Check sheet for the drawn part. Datum: minimum x, y, z corner. Units: mm. Give positions to 0.01 mm unless a question says otherwise; leave off trailing zeros. Order: outer loops, then holes, each group sorted by start corner. A loop starts at its lowest first (then second) coordinate and runs counter-clockwise, first axis right, second up.
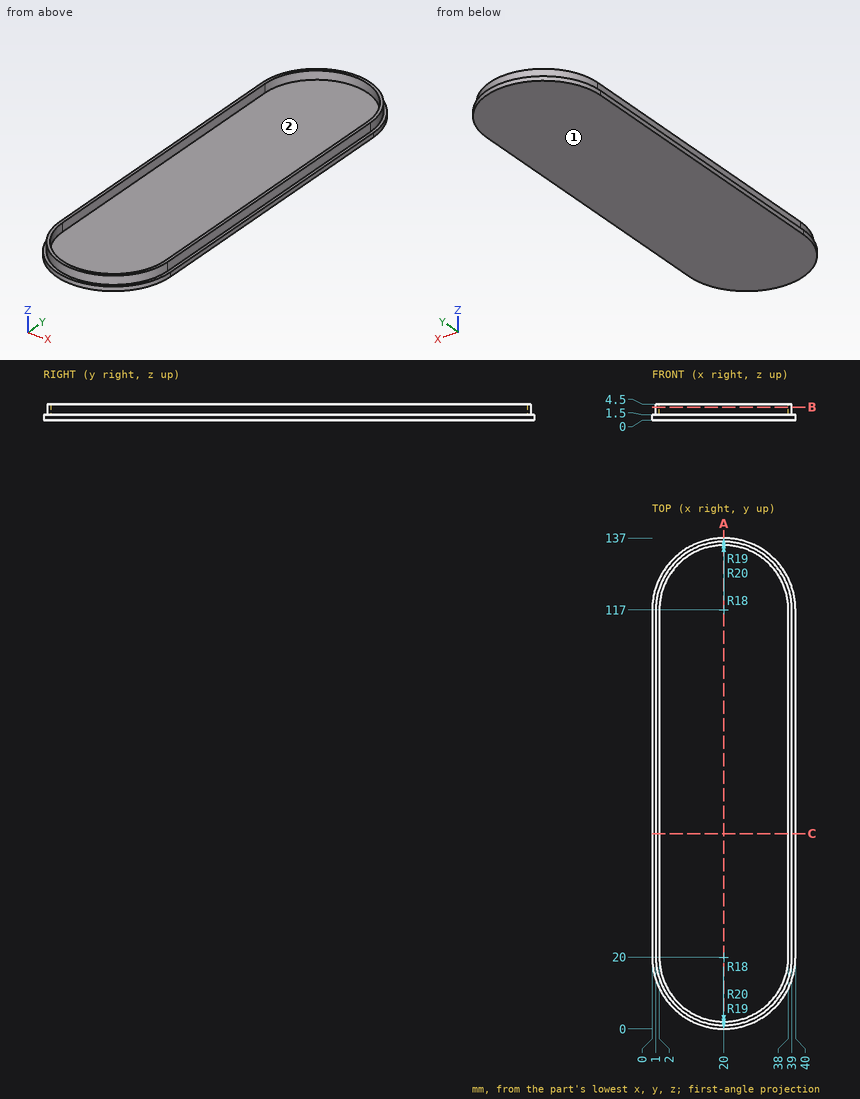
Item 1: Sectioned sample at B-B (z = 3.6). Enter the section's corners in (x, y), and give its area (3 significant figures).
Reported:
outline: (1, 20) arc R19 ccw to (39, 20) - (39, 117) arc R19 ccw to (1, 117) - close; hole (2, 20) arc R18 ccw to (38, 20) - (38, 117) arc R18 ccw to (2, 117) - close
area: 310 mm2
Item 2: Draft check along Y on the marked faces 1 and 2. Enter one of: released by +Y, released by -Y, zero draft, split by the parting line, or undercut.
Reported:
face 1: zero draft
face 2: undercut
Item 3: Scan lines: L1, parallel to X at y = 110.5, z = 2.05; L2, parallel to Z at x = 24, y = 118; L3, parallel to Y at x = 26.5, z = 3.8. Record each from-to range of solid material in increasing order.
Reported:
L1: x = 1 to 2, 38 to 39
L2: z = 0 to 1.5
L3: y = 2.15 to 3.21, 133.79 to 134.85
Item 4: Gauge pin test, flat ends, axial feed: pin 1 (1.5 mm diameter, centred on y = 72, z = 3.5, fed in from +X); pin 2 (12 mm diameter, centred on x = 14, y = 43.5, fed in from +Z); pin 3 (0.9 mm diameter, centred on y = 86, z = 2.5, fed in from -X). Record the tip position at first contact, or that the pin passes through.
Reported:
pin 1: stops at x = 39
pin 2: stops at z = 1.5
pin 3: stops at x = 1
Item 5: Sectioned sample at A-A (x = 20). Enter the section's corners in (y, z), and give its area (4 significant figures).
Reported:
outline: (0, 0) - (137, 0) - (137, 1.5) - (136, 1.5) - (136, 4.5) - (135, 4.5) - (135, 1.5) - (2, 1.5) - (2, 4.5) - (1, 4.5) - (1, 1.5) - (0, 1.5) - close
area: 211.5 mm2
Item 6: Sectioned sample at C-C (y = 54.5). Enter the section's corners in (x, z), and give its area (3 significant figures).
Reported:
outline: (0, 0) - (40, 0) - (40, 1.5) - (39, 1.5) - (39, 4.5) - (38, 4.5) - (38, 1.5) - (2, 1.5) - (2, 4.5) - (1, 4.5) - (1, 1.5) - (0, 1.5) - close
area: 66.0 mm2
